Read the model definition and answer for the solid it produces. Units are mm, in the model's axes. A direction names the side the tool comes from. Coordinates: 2 decimals unless noted, no trailing zeros. Loops run counter-clockwise (first coordinate to the right, second up) from the corner with the lowest first, then second, coordinate; pieces in that order, holes last. Notation, with made-up numbers: (-13.75, 68) -> (31.25, 68) arc R15 ccw to (31.25, 97) -> close; hole circle Ø11 at (-14.75, 87). An arc over 180 degrees is marked (long way). Answer as a JSON object with one key per item and string values. Group by question number.
1) Consider probe 1 along Z at (x, y) = (3.75, 54.8); probe 2 along X at (y, z) = (39.5, 11); probe 3 along Z at (x, y) = (122, 47.5). Determine where each line is inside the solid, lowest interval first. Write a range as [from, to].
2) Section B-B, the plane z = 6.5 is taken. Give the vertices of the cut face in (x, y).
3) Section A-A, the plane y = 49 is taken. Give the vertices of the cut face in (x, z).
4) Determine the mould class of faces 6 (the face through (99, 29, 80)), 7 (the face through (99, 29, 77.5)), 8 (the face through (99, 0, 39)) for opening direction Z: released by +Z, released by -Z, zero draft, split by the parting line, or undercut.
5) Section D-D, the plane z = 58.5 is taken. Give the vertices of the cut face in (x, y), plus the area to 3 significant figures.
6) Section C-C, the plane x = 149.5 is taken. Give the vertices of the cut face in (y, z).
7) Flat-ended cylindrical pins translate along their axes: P1, Ø3, axis at y = 1, z = 43, coming from the -X side; P2, Ø1.6, axis at x = 124, y = 56, coming from the +Z side; P3, Ø10, axis at x = 150.5, y = 45, coming from the -Z side; P4, Ø8, axis at x = 25, z = 70.5, coming from the -Y side. Find the tip coordinate at first contact, or state that the pin passes through.
8) Which of the six approach directions +Z, -Z, +X, -X, +Y, -Y give full straight-line access (tool end or side, diameter ignored) to faces 1 (the face through (132, 60, 81)), 2 (the face through (68, 57.5, 4)), 3 (the face through (99, 29, 0)), 4 (the face through (200, 28, 39)), 5 (the face through (99, 29, 2.5))?
from build123d import *

# Parameters (mm, degrees)
SKETCH1_W            = 200
SKETCH1_H            = 60
BOSS_EXTRUDE1_DEPTH  = 80
SKETCH2_W            = 185
SKETCH2_H            = 75
CUT_EXTRUDE1_DEPTH   = 57.5
SKETCH3_W            = 7.5
SKETCH3_H            = 75
CUT_EXTRUDE2_DEPTH   = 2.5
SKETCH4_W            = 210
SKETCH4_H            = 2.5
BOSS_EXTRUDE7_DEPTH  = 10
SKETCH9_W            = 210
SKETCH9_H            = 2.5
BOSS_EXTRUDE8_DEPTH  = 10
SKETCH10_W           = 100
SKETCH10_H           = 2.5
BOSS_EXTRUDE9_DEPTH  = 10
SKETCH11_R           = 1.5
CUT_EXTRUDE3_DEPTH   = 5
SKETCH12_W           = 185
SKETCH12_H           = 2
BOSS_EXTRUDE11_DEPTH = 2
SKETCH13_W           = 185
SKETCH13_H           = 2
BOSS_EXTRUDE12_DEPTH = 2
SKETCH14_W           = 55
SKETCH14_H           = 2.5
CUT_EXTRUDE4_DEPTH   = 3
SKETCH15_W           = 25
SKETCH15_H           = 15
CUT_EXTRUDE5_DEPTH   = 2.5


with BuildPart() as part:
    # Sketch1 → Boss-Extrude1 (new body)
    with BuildSketch(Plane.XY):
        with Locations((100, 30)):
            Rectangle(SKETCH1_W, SKETCH1_H)
    extrude(amount=BOSS_EXTRUDE1_DEPTH)

    # Sketch2 → Cut-Extrude1 (cut)
    with BuildSketch(Plane(origin=(0, 60, 0), x_dir=(1, 0, 0), z_dir=(0, 1, 0))):
        with Locations((100, -40)):
            Rectangle(SKETCH2_W, SKETCH2_H)
    extrude(amount=-CUT_EXTRUDE1_DEPTH, mode=Mode.SUBTRACT)

    # Sketch3 → Cut-Extrude2 (cut)
    with BuildSketch(Plane(origin=(0, 60, 0), x_dir=(1, 0, 0), z_dir=(0, 1, 0))):
        with Locations((3.75, -40)):
            Rectangle(SKETCH3_W, SKETCH3_H)
    extrude(amount=-CUT_EXTRUDE2_DEPTH, mode=Mode.SUBTRACT)

    # Sketch4 → Boss-Extrude7 (add)
    with BuildSketch(Plane(origin=(0, 0, 0), x_dir=(-1, 0, 0), z_dir=(0, 0, -1))):
        with Locations((-95, 58.75)):
            Rectangle(SKETCH4_W, SKETCH4_H)
    extrude(amount=BOSS_EXTRUDE7_DEPTH)

    # Sketch9 → Boss-Extrude8 (add)
    with BuildSketch(Plane.XY.offset(80)):
        with Locations((95, 58.75)):
            Rectangle(SKETCH9_W, SKETCH9_H)
    extrude(amount=BOSS_EXTRUDE8_DEPTH)

    # Sketch10 → Boss-Extrude9 (add)
    with BuildSketch(Plane(origin=(200, 0, 0), x_dir=(0, 0, -1), z_dir=(1, 0, 0))):
        with Locations((-40, 58.75)):
            Rectangle(SKETCH10_W, SKETCH10_H)
    extrude(amount=BOSS_EXTRUDE9_DEPTH)

    # Sketch11 → Cut-Extrude3 (cut)
    with BuildSketch(Plane(origin=(0, 57.5, 0), x_dir=(1, 0, 0), z_dir=(0, 1, 0))):
        with Locations((3.75, -40.265298021)):
            Circle(SKETCH11_R)
    extrude(amount=-CUT_EXTRUDE3_DEPTH, mode=Mode.SUBTRACT)

    # Sketch12 → Boss-Extrude11 (add)
    with BuildSketch(Plane(origin=(0, 0, 77.5), x_dir=(-1, 0, 0), z_dir=(0, 0, -1))):
        with Locations((-100, 56.5)):
            Rectangle(SKETCH12_W, SKETCH12_H)
    extrude(amount=BOSS_EXTRUDE11_DEPTH)

    # Sketch13 → Boss-Extrude12 (add)
    with BuildSketch(Plane.XY.offset(2.5)):
        with Locations((100, 56.5)):
            Rectangle(SKETCH13_W, SKETCH13_H)
    extrude(amount=BOSS_EXTRUDE12_DEPTH)

    # Sketch14 → Cut-Extrude4 (cut)
    with BuildSketch(Plane.ZY.offset(-192.5)):
        with Locations((40, 56.25)):
            Rectangle(SKETCH14_W, SKETCH14_H)
    extrude(amount=-CUT_EXTRUDE4_DEPTH, mode=Mode.SUBTRACT)

    # Sketch15 → Cut-Extrude5 (cut)
    with BuildSketch(Plane(origin=(0, 2.5, 0), x_dir=(1, 0, 0), z_dir=(0, 1, 0))):
        with Locations((30, -40)):
            Rectangle(SKETCH15_W, SKETCH15_H)
    extrude(amount=-CUT_EXTRUDE5_DEPTH, mode=Mode.SUBTRACT)


solid = part.part
Determined:
{
 "1": {"probe 1": "[0, 38.77], [41.77, 80]", "probe 2": "[0, 7.5], [192.5, 200]", "probe 3": "[0, 2.5], [77.5, 80]"},
 "2": {"outline": "(0, 0) -> (200, 0) -> (200, 57.5) -> (210, 57.5) -> (210, 60) -> (192.5, 60) -> (192.5, 2.5) -> (7.5, 2.5) -> (7.5, 57.5) -> (0, 57.5) -> close"},
 "3": {"outline": "(0, 0) -> (200, 0) -> (200, 80) -> (0, 80) -> close; hole (7.5, 2.5) -> (192.5, 2.5) -> (192.5, 77.5) -> (7.5, 77.5) -> close"},
 "4": {"face 6": "released by +Z", "face 7": "undercut", "face 8": "zero draft"},
 "5": {"outline": "(0, 0) -> (200, 0) -> (200, 57.5) -> (210, 57.5) -> (210, 60) -> (192.5, 60) -> (192.5, 57.5) -> (195.5, 57.5) -> (195.5, 55) -> (192.5, 55) -> (192.5, 2.5) -> (7.5, 2.5) -> (7.5, 57.5) -> (0, 57.5) -> close", "area": "1,360 mm²"},
 "6": {"outline": "(0, 0) -> (57.5, 0) -> (57.5, -10) -> (60, -10) -> (60, 2.5) -> (57.5, 2.5) -> (57.5, 4.5) -> (55.5, 4.5) -> (55.5, 2.5) -> (2.5, 2.5) -> (2.5, 77.5) -> (55.5, 77.5) -> (55.5, 75.5) -> (57.5, 75.5) -> (57.5, 77.5) -> (60, 77.5) -> (60, 90) -> (57.5, 90) -> (57.5, 80) -> (0, 80) -> close"},
 "7": {"P1": "x = 0", "P2": "z = 80", "P3": "z = 0", "P4": "y = 0"},
 "8": {"face 1": "+Z, -Z, +X, -X, +Y", "face 2": "-X, +Y", "face 3": "-Z, +X, -X, -Y", "face 4": "+Z, -Z, +X, -Y", "face 5": "none"}
}
